Here's how the part is built. I have some questions about the finished solid (model axes, mm). A direction names the side the tool comes from. Round coordinates to 2 decimals unless told otherwise and drop trailing zeros. Loops run counter-clockwise (first coordinate to the right, second up) from the corner with the lowest first, then second, coordinate; pieces in that order, holes last. Notation, with made-up numbers: (21.5, 56.5) -> (59.5, 56.5) arc R31 cw to (59.5, 86.5) -> close; hole circle Ø1 at (43, 30). An arc over 180 degrees is marked (long way). Use one line per item in the form item = value. Start each with the question number.
Item 1: I'm going to push flat-ended pins straight in: pin 1 Ø2.5 at (x, z) = (-19.5, -4.5) entering from +Y; pin 2 Ø9 at (x, z) = (-5, -2.5) entering from +Y; pin 3 Ø2 at (x, z) = (-13.75, 0) entering from -Y; pin 4 Ø2 at (x, z) = (10, -2) entering from +Y. Where does each tip first touch, or does it pass through?
Item 2: If I drill on L1, parallel to X at y = -2.5, z = 0; L2, parallel to Z at x = 9.5, y = -3.5; L3, parallel to Y at x = -20, z = 5.25, over which ranges is the centre line in solid material (lowest first)? Write a range as [from, to].
Item 3: If we section it at B-B (z = 0): Write out the boundary of the cut face in (x, y), then the cut area to 3 significant figures.
Item 4: Thinking about a two-plate mould opening in X: for faces 1 (the face through (-22, 8, 0)), 2 (the face through (6, -14.8, 0)), 3 (the face through (-3, -3, -9)), which applies, released by +X, released by -X, zero draft, split by the parting line, or undercut?
Item 5: If we section it at A-A (x = -13.75): Write out the boundary of the cut face in (y, z), then the cut area to 3 significant figures.
Item 6: For faces 4 (the face through (-11.6, -10, 8)), 5 (the face through (-19.5, 14.8, 4.5)), 6 (the face through (0.62, -16.83, -1.08)), 7 (the face through (16.5, -5, 0)), 8 (the face through (-17, 15, 0)), which set-ups out of +Z, -Z, +X, -X, +Y, -Y let a thin tool reach every point of the face, with its end or its side?
Item 7: If we section it at C-C (y = 17.5): Write out the boundary of the cut face in (x, z).
Item 8: If we section it at D-D (x = 5.5): Write out the boundary of the cut face in (y, z), then the cut area to 3 significant figures.
```python
from build123d import *

# Parameters (mm, degrees)
SKETCH1_W               = 38.5
SKETCH1_H               = 19.45
BOSS_EXTRUDE1_DEPTH     = 9
SKETCH2_W               = 5
SKETCH2_H               = 19.65
BOSS_EXTRUDE2_DEPTH     = 9
SKETCH3_R               = 7.5
BOSS_EXTRUDE3_DEPTH     = 4.5
SKETCH4_W               = 23.2
SKETCH4_H               = 13
CUT_EXTRUDE1_DEPTH      = 17.45
SKETCH5_R               = 5
CUT_EXTRUDE3_DEPTH      = 4
CUT_EXTRUDE4_DEPTH      = 35.351710292
CUT_EXTRUDE4_DEPTH_BACK = 35.351710292
SKETCH6_W               = 10.4
SKETCH6_H               = 4
SKETCH7_R               = 0.8
CUT_EXTRUDE5_DEPTH      = 8
SKETCH8_R               = 0.8
CUT_EXTRUDE6_DEPTH      = 8
SKETCH9_R               = 0.8
CUT_EXTRUDE7_DEPTH      = 10
SKETCH10_R              = 0.8
CUT_EXTRUDE8_DEPTH      = 10


with BuildPart() as part:
    # Sketch1 → Boss-Extrude1 (new, symmetric)
    with BuildSketch(Plane.XY):
        with Locations((-2.75, -4.575)):
            Rectangle(SKETCH1_W, SKETCH1_H)
    extrude(amount=BOSS_EXTRUDE1_DEPTH, both=True)

    # Sketch2 → Boss-Extrude2 (add, symmetric)
    with BuildSketch(Plane.XY):
        with Locations((-19.5, 14.975)):
            Rectangle(SKETCH2_W, SKETCH2_H)
    extrude(amount=BOSS_EXTRUDE2_DEPTH, both=True)

    # Sketch3 → Boss-Extrude3 (add)
    with BuildSketch(Plane(origin=(0, -18.8, 0), x_dir=(1, 0, 0), z_dir=(0, 1, 0))):
        with Locations(Location((5.5, 0, 0), (0, 0, 270))):
            Circle(SKETCH3_R)
    extrude(amount=BOSS_EXTRUDE3_DEPTH)

    # Sketch4 → Cut-Extrude1 (cut)
    with BuildSketch(Plane(origin=(0, 5.15, 0), x_dir=(1, 0, 0), z_dir=(0, 1, 0))):
        Rectangle(SKETCH4_W, SKETCH4_H)
    extrude(amount=-CUT_EXTRUDE1_DEPTH, mode=Mode.SUBTRACT)

    # Sketch5 → Cut-Extrude3 (cut)
    with BuildSketch(Plane(origin=(0, -18.8, 0), x_dir=(1, 0, 0), z_dir=(0, 1, 0))):
        with Locations(Location((5.5, 0, 0), (0, 0, 270))):
            Circle(SKETCH5_R)
    extrude(amount=CUT_EXTRUDE3_DEPTH, mode=Mode.SUBTRACT)

    # Sketch6 → Cut-Extrude4 (cut, two sides: drawn at the far end of the back side and taken through both)
    with BuildSketch(Plane.XY.offset(-CUT_EXTRUDE4_DEPTH_BACK)):
        with Locations((-16.8, -10.3)):
            Rectangle(SKETCH6_W, SKETCH6_H)
    extrude(amount=CUT_EXTRUDE4_DEPTH + CUT_EXTRUDE4_DEPTH_BACK, mode=Mode.SUBTRACT)

    # Sketch7 → Cut-Extrude5 (cut)
    with BuildSketch(Plane(origin=(0, 5.15, 0), x_dir=(1, 0, 0), z_dir=(0, 1, 0))):
        with Locations(Location((-13.75, 0, 0), (0, 0, 270))):
            Circle(SKETCH7_R)
    extrude(amount=-CUT_EXTRUDE5_DEPTH, mode=Mode.SUBTRACT)

    # Sketch8 → Cut-Extrude6 (cut)
    with BuildSketch(Plane(origin=(0, 5.15, 0), x_dir=(1, 0, 0), z_dir=(0, 1, 0))):
        with Locations(Location((13.75, 0, 0), (0, 0, 270))):
            Circle(SKETCH8_R)
    extrude(amount=-CUT_EXTRUDE6_DEPTH, mode=Mode.SUBTRACT)

    # Sketch9 → Cut-Extrude7 (cut)
    with BuildSketch(Plane(origin=(0, 24.8, 0), x_dir=(1, 0, 0), z_dir=(0, 1, 0))):
        with Locations(Location((-19.5, -4.5, 0), (0, 0, 270))):
            Circle(SKETCH9_R)
    extrude(amount=-CUT_EXTRUDE7_DEPTH, mode=Mode.SUBTRACT)

    # Sketch10 → Cut-Extrude8 (cut)
    with BuildSketch(Plane(origin=(0, 24.8, 0), x_dir=(1, 0, 0), z_dir=(0, 1, 0))):
        with Locations(Location((-19.5, 4.5, 0), (0, 0, 270))):
            Circle(SKETCH10_R)
    extrude(amount=-CUT_EXTRUDE8_DEPTH, mode=Mode.SUBTRACT)


solid = part.part
```
Values found:
q1.pin_1 = 24.8
q1.pin_2 = 5.15
q1.pin_3 = -14.3
q1.pin_4 = -12.3
q2.L1 = [-22, -14.55], [-12.95, -11.6], [11.6, 12.95], [14.55, 16.5]
q2.L2 = [-9, -6.5], [6.5, 9]
q2.L3 = [-14.3, -12.3], [-8.3, 24.8]
q3.outline = (-22, -14.3) -> (-2, -14.3) -> (-2, -18.8) -> (0.5, -18.8) -> (0.5, -14.8) -> (10.5, -14.8) -> (10.5, -18.8) -> (13, -18.8) -> (13, -14.3) -> (16.5, -14.3) -> (16.5, 5.15) -> (14.55, 5.15) -> (14.55, -2.85) -> (12.95, -2.85) -> (12.95, 5.15) -> (11.6, 5.15) -> (11.6, -12.3) -> (-22, -12.3) -> close; (-22, -8.3) -> (-11.6, -8.3) -> (-11.6, 5.15) -> (-12.95, 5.15) -> (-12.95, -2.85) -> (-14.55, -2.85) -> (-14.55, 5.15) -> (-17, 5.15) -> (-17, 24.8) -> (-22, 24.8) -> close
q3.area = 403 mm2
q4.face_1 = released by -X
q4.face_2 = undercut
q4.face_3 = zero draft
q5.outline = (-14.3, -9) -> (-12.3, -9) -> (-12.3, 9) -> (-14.3, 9) -> close; (-8.3, -9) -> (5.15, -9) -> (5.15, -0.8) -> (-2.85, -0.8) -> (-2.85, 0.8) -> (5.15, 0.8) -> (5.15, 9) -> (-8.3, 9) -> close
q5.area = 265 mm2
q6.face_4 = +Z, -Z, -X
q6.face_5 = +Y
q6.face_6 = -Y
q6.face_7 = +Z, -Z, +X, +Y, -Y
q6.face_8 = +Z, -Z, +X, +Y
q7.outline = (-22, -9) -> (-17, -9) -> (-17, 9) -> (-22, 9) -> close; hole circle Ø1.6 at (-19.5, -4.5); hole circle Ø1.6 at (-19.5, 4.5)
q8.outline = (-18.8, -7.5) -> (-14.3, -7.5) -> (-14.3, -9) -> (5.15, -9) -> (5.15, -6.5) -> (-12.3, -6.5) -> (-12.3, 6.5) -> (5.15, 6.5) -> (5.15, 9) -> (-14.3, 9) -> (-14.3, 7.5) -> (-18.8, 7.5) -> (-18.8, 5) -> (-14.8, 5) -> (-14.8, -5) -> (-18.8, -5) -> close
q8.area = 151 mm2
